The model under review builds one solid part; all positions refer to its coordinate system, in mm. A direction names the side the tool comes from. Coordinates: 2 decimals unless noted, no trailing zeros. Write each loop counter-clockwise with the first axis right and the second up, starting at its lowest first coordinate (ties: lowest second). Pieces come first, ordered by that corner, then holes. Notation, with made-up numbers: (12.5, 44.25) - (25.5, 44.25) arc R31 ccw to (25.5, 77.25) - close; hole circle Ø6 at (54, -5). An arc over 180 degrees is marked (long way). Put each result on its own line as item: value. Start each with the question number.
Item 1: Mouldability with a two-part tool opening along Z and no side actions: class faces 4 (the face through (1, -10, -16)), 5 (the face through (7.16, -4.55, -6.98)), 6 (the face through (11.138, -1.972, -0.507)), 7 (the face through (19.054, -6.958, -8.344)) as pulls with the +Z half, pulls with the -Z half, needs draft (parallel to the pull), parting line crosses it, or undercut.
Item 2: To check wall thickness, follow L1, parallel to X at y = -0.5, z = 1; L2, parallel to Z at x = 22, y = -2.8; L3, parallel to Z at x = 2.5, y = -8.25. State the ranges of each line that lie inside material, in increasing order. Write a range as [from, to].
Item 3: Consider section C-C on x = 22. Give the boundary of the cut face in (y, z), then the cut area to 3 significant figures.
Item 4: Consider section D-D on z = -26.5. Give the boundary of the cut face in (x, y), then the cut area to 3 significant figures.
Item 5: Consider section A-A on y = -8.5. Give the boundary of the cut face in (x, z).
Item 6: Consider section B-B on x = 0. Give the boundary of the cut face in (y, z), then the cut area to 3 significant figures.
Item 7: For pin 1 (5 mm diameter, centred on y = -8.5, z = -15.5, fed in from +X); pin 2 (6.5 mm diameter, centred on x = 3.5, z = -1.5, fed in from -Y); pin 3 (1.5 mm diameter, centred on y = -1, z = -10.5, fed in from +X); pin 4 (3 mm diameter, centred on x = 18, z = -14, fed in from -Y), all flat-tipped, find the tip position at first contact; note any pin that passes through.
Item 8: Machinability: for faces 1 (the face through (5.73, -6.96, -5.58)), 2 (the face through (-5.5, -9, -29.7)), 3 (the face through (11.79, -1.97, -17.83)), which of the approach directions +Z, -Z, +X, -X, +Y, -Y give a long, thin tool a straight path to every point of the face, cutting with its end or side? Answer none if there is none.
```python
from build123d import *

# Parameters (mm, degrees)
F1_DEPTH = 4
F3_DEPTH = 6
F5_DEPTH = 2
F7_DEPTH = 7
F8_R     = 1.5
F9_DEPTH = 10.001


with BuildPart() as f1:
    # F0 (on Front) → F1 (new body)
    with BuildSketch(Plane.XZ):
        with BuildLine():
            ThreePointArc((20.263158, 2.446095), (11, -0.508067), (1.736842, 2.446095))
            ThreePointArc((1.736842, 2.446095), (-2.082163, 2.159767), (-2.507986, -1.64621))
            ThreePointArc((-2.507986, -1.64621), (0.593406, -15.288544), (-6.004354, -27.62554))
            ThreePointArc((-6.004354, -27.62554), (-6.26024, -30.354478), (-3.551962, -30.776156))
            ThreePointArc((-3.551962, -30.776156), (11.985415, -17.624993), (24.537749, -1.599947))
            ThreePointArc((24.537749, -1.599947), (24.062275, 2.178767), (20.263158, 2.446095))
        make_face()
    extrude(amount=F1_DEPTH)

    # F2 (on face) → F3 (join)
    with BuildSketch(Plane.XZ.offset(4)):
        with BuildLine():
            ThreePointArc((7.754053, -1.968417), (5.68946, -5.624059), (2.057931, -7.730777))
            ThreePointArc((2.057931, -7.730777), (0.908195, -8.554249), (0.590568, -9.932333))
            ThreePointArc((0.590568, -9.932333), (-0.487406, -19.606222), (-6.004354, -27.62554))
            ThreePointArc((-6.004354, -27.62554), (-6.26024, -30.354478), (-3.551962, -30.776156))
            ThreePointArc((-3.551962, -30.776156), (8.352605, -21.210498), (18.661792, -9.94368))
            ThreePointArc((18.661792, -9.94368), (19.049057, -8.320033), (18.069983, -6.968139))
            ThreePointArc((18.069983, -6.968139), (15.645578, -4.860177), (14.245947, -1.968417))
            ThreePointArc((14.245947, -1.968417), (13.477217, -0.838298), (12.162164, -0.465804))
            ThreePointArc((12.162164, -0.465804), (11, -0.508067), (9.837836, -0.465804))
            ThreePointArc((9.837836, -0.465804), (8.522783, -0.838298), (7.754053, -1.968417))
        make_face()
    extrude(amount=F3_DEPTH)

    # F4 (on face) → F5 (cut)
    with BuildSketch(Plane.XZ.offset(10)):
        with BuildLine():
            ThreePointArc((1.581491, -9.797902), (0.449618, -19.955486), (-5.343177, -28.37577))
            ThreePointArc((-5.343177, -28.37577), (-5.47112, -29.740239), (-4.116981, -29.951078))
            ThreePointArc((-4.116981, -29.951078), (7.66854, -20.481077), (17.874636, -9.326927))
            ThreePointArc((17.874636, -9.326927), (18.068268, -8.515104), (17.578731, -7.839157))
            ThreePointArc((17.578731, -7.839157), (14.851275, -5.467699), (13.276691, -2.214469))
            ThreePointArc((13.276691, -2.214469), (12.892325, -1.649409), (12.234799, -1.463162))
            ThreePointArc((12.234799, -1.463162), (11, -1.508067), (9.765201, -1.463162))
            ThreePointArc((9.765201, -1.463162), (9.107675, -1.649409), (8.723309, -2.214469))
            ThreePointArc((8.723309, -2.214469), (6.400643, -6.327067), (2.315173, -8.697125))
            ThreePointArc((2.315173, -8.697125), (1.740304, -9.108861), (1.581491, -9.797902))
        make_face()
    extrude(amount=-F5_DEPTH, mode=Mode.SUBTRACT)

    # F6 (on face) → F7 (cut)
    with BuildSketch(Plane.XZ.offset(8)):
        with BuildLine():
            ThreePointArc((-4.682, -29.126), (6.984475, -19.751655), (17.087479, -8.710174))
            ThreePointArc((17.087479, -8.710174), (14.056973, -6.075221), (12.307434, -2.460521))
            ThreePointArc((12.307434, -2.460521), (11, -2.508067), (9.692566, -2.460521))
            ThreePointArc((9.692566, -2.460521), (7.111825, -7.030074), (2.572414, -9.663472))
            ThreePointArc((2.572414, -9.663472), (1.386642, -20.30475), (-4.682, -29.126))
        make_face()
    extrude(amount=-F7_DEPTH, mode=Mode.SUBTRACT)

    # F8 (on Front) → F9 (cut, through all)
    with BuildSketch(Plane.XZ):
        Circle(F8_R)
        with Locations((22, 0)):
            Circle(F8_R)
    extrude(amount=F9_DEPTH, mode=Mode.SUBTRACT)


solid = f1.part
```
Report:
1. face 4: needs draft
1. face 5: undercut
1. face 6: pulls with the +Z half
1. face 7: parting line crosses it
2. L1: [-2.83, -1.12], [1.12, 4.22], [17.78, 20.88], [23.12, 24.83]
2. L2: [-5.43, -1.5], [1.5, 3]
2. L3: [-26.29, -25], [-8.65, -7.6]
3. outline: (-4, -5.43) - (0, -5.43) - (0, -1.5) - (-4, -1.5) - close; (-4, 1.5) - (0, 1.5) - (0, 3) - (-4, 3) - close
3. area: 21.7 mm²
4. outline: (-4.83, -10) - (-3.47, -10) - (-3.47, -8) - (-2.16, -8) - (-2.16, -1) - (-1.03, -1) - (-1.03, -8) - (0.62, -8) - (0.62, -10) - (2.23, -10) - (2.23, 0) - (-4.83, 0) - close
4. area: 54.6 mm²
5. outline: (-6, -27.63) arc R2 ccw to (-3.55, -30.78) arc R100 ccw to (18.66, -9.94) arc R2 ccw to (18.07, -6.97) arc R8 cw to (14.25, -1.97) arc R2 ccw to (12.16, -0.47) arc R16 cw to (9.84, -0.47) arc R2 ccw to (7.75, -1.97) arc R8 cw to (2.06, -7.73) arc R2 ccw to (0.59, -9.93) arc R20 cw to start; hole (-5.34, -28.38) arc R1 ccw to (-4.12, -29.95) arc R99 ccw to (17.87, -9.33) arc R1 ccw to (17.58, -7.84) arc R9 cw to (13.28, -2.21) arc R1 ccw to (12.23, -1.46) arc R17 cw to (9.77, -1.46) arc R1 ccw to (8.72, -2.21) arc R9 cw to (2.32, -8.7) arc R1 ccw to (1.58, -9.8) arc R21 cw to start
6. outline: (-10, -28.23) - (0, -28.23) - (0, -18.12) - (-10, -18.12) - (-10, -21.06) - (-8, -21.06) - (-8, -23.31) - (-1, -23.31) - (-1, -25.71) - (-8, -25.71) - (-8, -26.97) - (-10, -26.97) - close; (-4, -7.12) - (0, -7.12) - (0, -1.5) - (-4, -1.5) - close; (-4, 1.5) - (0, 1.5) - (0, 3) - (-4, 3) - close
6. area: 101 mm²
7. pin 1: x = 16.17
7. pin 2: y = -4
7. pin 3: x = 18.81
7. pin 4: through
8. face 1: +Z, -X, -Y
8. face 2: -Y
8. face 3: -Z, +X, +Y, -Y
